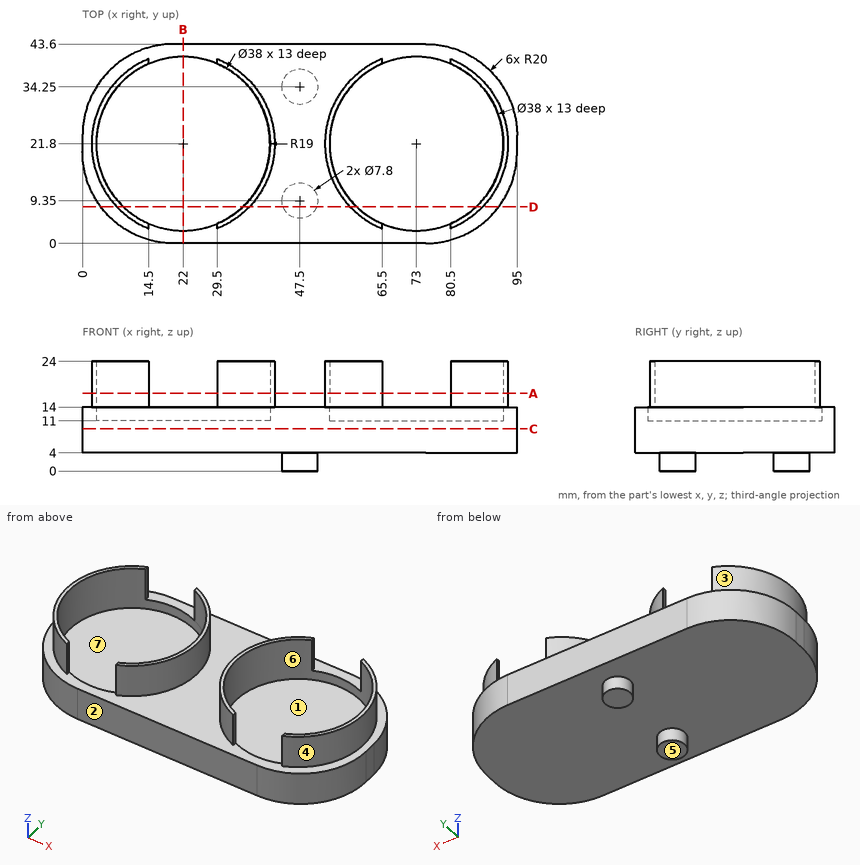
Source: three-view drawing plus pictorial views. Frame: mm from the lowest corner of the part. A direction names the side the tool comes from. Give positions to 0.01 mm unless a question says otherwise; leave off trailing zeros. Write each loop counter-clockwise with the first axis right and the second up, starting at its lowest first coordinate (ties: lowest second). Pieces come first, ordered by that corner, then holes. Notation, with made-up numbers: (75.25, -14.5) -> (106.25, -14.5) arc R11 ccw to (106.25, 2.5) -> close; hole circle Ø1 at (73, 29). An arc over 180 degrees is marked (long way). Answer in a Markdown table with one row per item.
(1) Ray query, line 1 along Z through (x, y) = (10, 29); line 2 along X through (y, z) = (32.5, 12.5); line 3 along X through (y, z) = (32.5, 19.25). Return the intervals inside material, ascending. Write a range as [from, to].
Answers below:
| item | result |
|---|---|
| line 1 | [4, 11] |
| line 2 | [2.09, 6.3], [37.7, 57.3], [88.7, 92.91] |
| line 3 | [5.1, 6.3], [37.7, 38.9], [56.1, 57.3], [88.7, 89.9] |
(2) Section query B-B on x = 22. Return loops of the section in (y, z), then the cut area to 3 significant figures.
Answers below:
| item | result |
|---|---|
| outline | (0, 4) -> (43.6, 4) -> (43.6, 14) -> (40.8, 14) -> (40.8, 11) -> (2.8, 11) -> (2.8, 14) -> (0, 14) -> close |
| area | 322 mm^2 |
(3) Section query D-D on y = 8. Return loops of the section in (x, z).
Answers below:
| item | result |
|---|---|
| outline | (4, 4) -> (43.84, 4) -> (43.84, 0) -> (51.16, 0) -> (51.16, 4) -> (91, 4) -> (91, 14) -> (87.48, 14) -> (87.48, 24) -> (86.06, 24) -> (86.06, 11) -> (59.94, 11) -> (59.94, 24) -> (58.52, 24) -> (58.52, 14) -> (36.48, 14) -> (36.48, 24) -> (35.06, 24) -> (35.06, 11) -> (8.94, 11) -> (8.94, 24) -> (7.52, 24) -> (7.52, 14) -> (4, 14) -> close |
(4) Pin query (flat end, axial travel): pin 1 (1 mm diameter, centred on x = 25.5, z = 15, fed in from +Y); pin 2 (1.2 mm diameter, centred on y = 40, z = 18, fed in from +X); pin 3 (8 mm diameter, centred on x = 55, y = 10, fed in from +Z); pin 4 (0.5 mm diameter, centred on y = 39.5, z = 18.5, fed in from -X). Return the tip coordinate at first contact, or that it passes through.
Answers below:
| item | result |
|---|---|
| pin 1 | through |
| pin 2 | x = 82.5 |
| pin 3 | z = 24 |
| pin 4 | x = 12.23 |
(5) Set-up query: the marked faces 1, 2 and 3. Return all of +Z, -Z, +X, -X, +Y, -Y with unobstructed straight access to the full face (end or side cutting, diameter ignored); none if empty.
Answers below:
| item | result |
|---|---|
| face 1 | +Z |
| face 2 | +Z, -Z, +X, -X, -Y |
| face 3 | +Z, -X |
(6) Section query A-A on z = 17. Return loops of the section in (x, y), then the cut area to 3 significant figures.
Answers below:
| item | result |
|---|---|
| outline | (14.5, 3.26) -> (14.5, 4.34) arc R19 cw to (14.5, 39.26) -> (14.5, 40.34) arc R20 ccw to start; (29.5, 3.26) arc R20 ccw to (29.5, 40.34) -> (29.5, 39.26) arc R19 cw to (29.5, 4.34) -> close; (65.5, 3.26) -> (65.5, 4.34) arc R19 cw to (65.5, 39.26) -> (65.5, 40.34) arc R20 ccw to start; (80.5, 3.26) arc R20 ccw to (80.5, 40.34) -> (80.5, 39.26) arc R19 cw to (80.5, 4.34) -> close |
| area | 183 mm^2 |
(7) Draft query along Y for the marked faces 4, 5, 6 and 7. Return one class per face: +Y half, -Y half, draft (parallel to the pull), parting line (faces both ways), or undercut.
Answers below:
| item | result |
|---|---|
| face 4 | parting line |
| face 5 | draft |
| face 6 | undercut |
| face 7 | undercut |
(8) Section query C-C on z = 9.25. Return loops of the section in (x, y).
Answers below:
| item | result |
|---|---|
| outline | (0, 20) arc R20 ccw to (20, 0) -> (75, 0) arc R20 ccw to (95, 20) -> (95, 23.6) arc R20 ccw to (75, 43.6) -> (20, 43.6) arc R20 ccw to (0, 23.6) -> close |
